Model file for the job. Use its own axes, mm. A direction names the side the tool comes from. Round coordinates to 2 decimals unless told otherwise and drop trailing zeros. Order: outer loops, then holes, each group sorted by start corner. A loop starts at its lowest first (then second) coordinate and runs counter-clockwise, first axis right, second up. Notation, with made-up numbers: (41.25, 39.25) - (70.25, 39.25) arc R31 cw to (70.25, 78.25) - close; hole circle Ø8 at (69.25, 87.5). An arc over 180 degrees is marked (long way). Use one line per item in the form item = value.
from build123d import *

# Parameters (mm, degrees)
SKETCH11_W              = 37.7
SKETCH11_H              = 28.7
SKETCH11_R              = 9.7
BOSS_EXTRUDE1_DEPTH     = 42
BOSS_EXTRUDE3_REACH     = 56.25
SKETCH15_W              = 37.7
SKETCH15_H              = 5
SKETCH12_R              = 4
CUT_EXTRUDE1_DEPTH      = 40
SKETCH23_W              = 20
SKETCH23_H              = 20
BOSS_EXTRUDE4_DEPTH     = 14.35
CUT_EXTRUDE2_DEPTH      = 49.220794396
CUT_EXTRUDE2_DEPTH_BACK = 49.220794396
SKETCH24_R              = 1.5
FILLET1_R               = 5


with BuildPart() as part:
    # Sketch11 → Boss-Extrude1 (new body)
    with BuildSketch(Plane(origin=(0, 0, 0), x_dir=(1, 0, 0), z_dir=(0, 1, 0))):
        Rectangle(SKETCH11_W, SKETCH11_H)
        with Locations(Location((0, 0, 0), (0, 0, 90))):
            Circle(SKETCH11_R, mode=Mode.SUBTRACT)
    extrude(amount=BOSS_EXTRUDE1_DEPTH)

    # Boss-Extrude3: up to this face of the body (flat: up to its plane)
    boss_extrude3_end = Plane(part.part.faces().sort_by_distance((0, 21, -14.35))[0])
    # Sketch15 → Boss-Extrude3 (add, up to the picked face)
    with BuildSketch(Plane.XY.offset(14.35), mode=Mode.PRIVATE) as boss_extrude3_sk1:
        with Locations((0, 2.5)):
            Rectangle(SKETCH15_W, SKETCH15_H)
    boss_extrude3_tool1 = split(extrude(boss_extrude3_sk1.sketch, amount=-BOSS_EXTRUDE3_REACH, mode=Mode.PRIVATE), bisect_by=boss_extrude3_end, keep=Keep.BOTH, mode=Mode.PRIVATE)
    add(boss_extrude3_tool1.solids().sort_by(Axis((0, 2.5, 14.35), (0, 0, -1)))[0])

    # Sketch12 → Cut-Extrude1 (cut)
    with BuildSketch(Plane(origin=(18.85, 0, 0), x_dir=(0, 0, -1), z_dir=(1, 0, 0))):
        with Locations((0, 33)):
            Circle(SKETCH12_R)
        with Locations((0, 17)):
            Circle(SKETCH12_R)
    extrude(amount=-CUT_EXTRUDE1_DEPTH, mode=Mode.SUBTRACT)

    # Sketch23 → Boss-Extrude4 (add, symmetric)
    with BuildSketch(Plane.XY):
        with Locations((0, -10)):
            Rectangle(SKETCH23_W, SKETCH23_H)
        with BuildLine():
            Line((-1.824828759, -7.525), (1.824828759, -7.525))
            ThreePointArc((1.824828759, -7.525), (0, -13.075), (-1.824828759, -7.525))
        make_face(mode=Mode.SUBTRACT)
    extrude(amount=BOSS_EXTRUDE4_DEPTH, both=True)

    # Sketch24 → Cut-Extrude2 (cut, two sides: drawn at the far end of the back side and taken through both)
    with BuildSketch(Plane(origin=(0, 0, 0), x_dir=(0, 0, -1), z_dir=(1, 0, 0)).offset(-CUT_EXTRUDE2_DEPTH_BACK)):
        with Locations((0, -10)):
            Circle(SKETCH24_R)
    extrude(amount=CUT_EXTRUDE2_DEPTH + CUT_EXTRUDE2_DEPTH_BACK, mode=Mode.SUBTRACT)

    # Fillet1
    fillet1_edges = [part.edges().sort_by_distance(p)[0] for p in [
        (10, 0, 0),
        (-10, 0, 0),
    ]]
    fillet(fillet1_edges, radius=FILLET1_R)


solid = part.part
(1) Slice it at A-A on x = 0. Give the cut face in (y, z) (3 decimals).
Report:
outline = (-20, -14.35) - (-13.075, -14.35) - (-13.075, 14.35) - (-20, 14.35) - close; (-7.525, -14.35) - (42, -14.35) - (42, -9.7) - (5, -9.7) - (5, 9.7) - (42, 9.7) - (42, 14.35) - (-7.525, 14.35) - close
(2) Slice it at D-D on y = -10. Give the cut face in (x, z) (3 decimals), then the cut area to 3 significant figures.
Report:
outline = (-10, -14.35) - (-3.075, -14.35) - (-3.075, -1.5) - (-10, -1.5) - close; (-10, 1.5) - (-3.075, 1.5) - (-3.075, 14.35) - (-10, 14.35) - close; (3.075, -14.35) - (10, -14.35) - (10, -1.5) - (3.075, -1.5) - close; (3.075, 1.5) - (10, 1.5) - (10, 14.35) - (3.075, 14.35) - close
area = 356 mm2
(3) Pin check, flat tips, straight feed: pin 1 (4 mm diameter, centred on y = -10, z = 0, fed in from -X); pin 2 (1.5 mm diameter, centred on x = -7, z = 0.5, fed in from +Y); pin 3 (12 mm diameter, centred on y = -16, z = -5, fed in from +X). Stop position of each tip, or through.
Report:
pin_1 = -10
pin_2 = 5
pin_3 = 10
(4) Probe probe 1 along Z at (x, y) = (-14, 17); probe 2 along X at (y, z) = (7.5, 0.25); probe 3 along Z at (x, y) = (4, 31). List the from-to ranges inside material, lowest first. Write a range as [from, to].
Report:
probe_1 = [-14.35, -4], [4, 14.35]
probe_2 = [-18.85, -9.7], [9.7, 18.85]
probe_3 = [-14.35, -8.84], [8.84, 14.35]
(5) Slice it at B-B on y = 33. Give the cut face in (x, z), then the cut area to 3 significant figures.
Report:
outline = (-18.85, -14.35) - (18.85, -14.35) - (18.85, -4) - (8.84, -4) arc R9.7 cw to (-8.84, -4) - (-18.85, -4) - close; (-18.85, 4) - (-8.84, 4) arc R9.7 cw to (8.84, 4) - (18.85, 4) - (18.85, 14.35) - (-18.85, 14.35) - close
area = 635 mm2
(6) Tool access for faces 5 (the face through (17, 0, 0)), 6 (the face through (-2.914, 23.241, -9.252)), 7 (the face through (0, -20, 0)), 8 (the face through (-17, 0, 0)), 9 (the face through (0, -7.525, 0)): list every direction of +Z, -Z, +X, -X, +Y, -Y with a clear straight run to the whole face (end or side of a thin tool).
Report:
face_5 = +Z, -Z, +X, -Y
face_6 = +Y
face_7 = +Z, -Z, +X, -X, -Y
face_8 = +Z, -Z, -X, -Y
face_9 = +Z, -Z
(7) Pull direction X, two halves, no side cores. Call faces 1 (the face through (0, 5, 0)), 2 (the face through (0, 17, -14.35)), 3 (the face through (-12, -1, 0)), 4 (the face through (10, -13, 0)): released by +X, released by -X, zero draft, split by the parting line, or undercut.
Report:
face_1 = undercut
face_2 = zero draft
face_3 = released by -X
face_4 = released by +X
(8) Slice it at C-C on z = -12.5. Give the cut face in (x, y) (3 decimals).
Report:
outline = (-18.85, 0) - (-15, 0) arc R5 cw to (-10, -5) - (-10, -20) - (10, -20) - (10, -5) arc R5 cw to (15, 0) - (18.85, 0) - (18.85, 42) - (-18.85, 42) - close; hole (-1.825, -7.525) arc R3.075 ccw (long way) to (1.825, -7.525) - close
